Work out the finished part from the listing and answer in its coordinate system (mm). A direction names the side the tool comes from. Give positions to 0.01 mm unless a question says otherwise; leave off trailing zeros. Write each loop counter-clockwise with the first axis right and the second up, starting at its lowest first coordinate (ties: lowest second). Pieces come first, ordered by that corner, then holes.
1) Find section B-B (z = 3.75). Determine the outline of the cut face in (x, y), plus the area to 3 significant figures.
2) A tool of negligible diameter and unlimited length cuts with its end or side. For faces 1 (the face through (10, 19, 0)), 2 (the face through (-1, 31, 2)), 3 (the face through (-5, 34.5, 0)), 4 (the face through (-13, 3, 2)), from which of +Z, -Z, +X, -X, +Y, -Y can it reach the whole face along a straight path? Write none if from no direction.
3) Straight lines are drawn through the part: probe 1 along X at (y, z) = (28.5, 5.5); probe 2 along Y at (x, z) = (1.5, 0.5); probe 3 along Y at (x, z) = (3.5, 0.5). For each, find the intervals that lie inside material, in ascending order.
4) Determine the mould class of faces 5 (the face through (-18.719, -0.212, 0.826)), 6 (the face through (0, 12, 7)), 7 (the face through (-21, 0, 0)) for opening direction Z: pulls with the +Z half, pulls with the -Z half, needs draft (parallel to the pull), parting line crosses it, or undercut.
5) Given pin 1 Ø4 at (y, z) = (23.5, -0.5) entering from -X; pin 2 Ø4 at (x, z) = (15, -2) entering from +Y; pin 3 Ø5 at (y, z) = (15, -3.5) entering from +X, each flat-ended and moving along its own axis, determine where each tip first touches the part or whether it passes through.
6) Find section C-C (x = -1.5). Count the separate pieces of the cut face and the enclosed holes in it, plus the area to 3 significant figures.
7) Find section A-A (y = 20). Determine the outline of the cut face in (x, z).
8) Find section D-D (x = -12). Determine the outline of the cut face in (y, z).
```python
from build123d import *

# Parameters (mm, degrees)
BOSS_EXTRUDE1_DEPTH     = 7
SKETCH2_R               = 2.75
CUT_EXTRUDE1_DEPTH      = 39.5
CUT_EXTRUDE2_DEPTH      = 42.512046444
CUT_EXTRUDE2_DEPTH_BACK = 42.512046444
SKETCH5_R               = 2
CHAMFER2_SIZE           = 0.5
FILLET2_R               = 0.5


with BuildPart() as part:
    # Sketch1 → Boss-Extrude1 (new, symmetric)
    with BuildSketch(Plane.XY):
        with BuildLine():
            Line((-21, -3), (-21, 3))
            Line((-21, 3), (-10, 3))
            Line((-10, 3), (-10, 34.5))
            Line((-10, 34.5), (-1, 34.5))
            Line((-1, 34.5), (-1, 25.916079783))
            ThreePointArc((-1, 25.916079783), (0, 14), (1, 25.916079783))
            Line((1, 25.916079783), (1, 34.5))
            Line((1, 34.5), (10, 34.5))
            Line((10, 34.5), (10, 3))
            Line((10, 3), (21, 3))
            Line((21, 3), (21, -3))
            Line((21, -3), (-21, -3))
        make_face()
    extrude(amount=BOSS_EXTRUDE1_DEPTH, both=True)

    # Sketch2 → Cut-Extrude1 (cut, through all)
    with BuildSketch(Plane(origin=(0, 3, 0), x_dir=(1, 0, 0), z_dir=(0, 1, 0))):
        with Locations(Location((15.904501915, 0, 0), (0, 0, 180))):
            Circle(SKETCH2_R)
        with Locations(Location((-16.095498085, 0, 0), (0, 0, 180))):
            Circle(SKETCH2_R)
    extrude(amount=-CUT_EXTRUDE1_DEPTH, mode=Mode.SUBTRACT)

    # Sketch5 → Cut-Extrude2 (cut, two sides: drawn at the far end of the back side and taken through both)
    with BuildSketch(Plane(origin=(-1, 0, 0), x_dir=(0, 0, -1), z_dir=(1, 0, 0)).offset(-CUT_EXTRUDE2_DEPTH_BACK)):
        with Locations((0.330734984, 30.208039892)):
            Circle(SKETCH5_R)
    extrude(amount=CUT_EXTRUDE2_DEPTH + CUT_EXTRUDE2_DEPTH_BACK, mode=Mode.SUBTRACT)

    # Chamfer2
    chamfer2_edges = [part.edges().sort_by_distance(p)[0] for p in [
        (0, 14, -7),
        (0, 14, 7),
        (18.654501915, 3, 0),
        (-13.345498085, 3, 0),
        (-10, 30.208039892, 1.669265016),
        (10, 30.208039892, 1.669265016),
    ]]
    chamfer(chamfer2_edges, length=CHAMFER2_SIZE)

    # Fillet2
    fillet2_edges = [part.edges().sort_by_distance(p)[0] for p in [
        (-15.5, 3, 7),
        (10, 18.75, -7),
        (15.5, 3, -7),
        (-21, 0, 7),
        (21, 0, -7),
        (-21, 0, -7),
        (-15.5, 3, -7),
        (-10, 18.75, -7),
        (21, 0, 7),
        (10, 34.5, 0),
        (21, 3, 0),
        (21, -3, 0),
        (-21, -3, 0),
        (-21, 3, 0),
        (-10, 34.5, 0),
        (15.5, 3, 7),
        (10, 18.75, 7),
        (-10, 18.75, 7),
    ]]
    fillet(fillet2_edges, radius=FILLET2_R)


solid = part.part
```
Results:
1. outline: (-21, -2.5) arc R0.5 ccw to (-20.5, -3) - (20.5, -3) arc R0.5 ccw to (21, -2.5) - (21, 2.5) arc R0.5 ccw to (20.5, 3) - (10, 3) - (10, 34) arc R0.5 ccw to (9.5, 34.5) - (1, 34.5) - (1, 25.92) arc R6 cw (long way) to (-1, 25.92) - (-1, 34.5) - (-9.5, 34.5) arc R0.5 ccw to (-10, 34) - (-10, 3) - (-20.5, 3) arc R0.5 ccw to (-21, 2.5) - close
1. area: 752 mm2
2. face 1: +Z, -Z, +X, +Y
2. face 2: +Z, -Z, +Y
2. face 3: +Z, -Z, +X, -X, +Y
2. face 4: +Z, -Z, -X, +Y
3. probe 1: x = -10 to -1, 1 to 10
3. probe 2: y = -3 to 14.19, 25.81 to 28.39, 32.03 to 34.5
3. probe 3: y = -3 to 15.13, 24.87 to 28.39, 32.03 to 34.5
4. face 5: undercut
4. face 6: pulls with the +Z half
4. face 7: needs draft
5. pin 1: stops at x = -10
5. pin 2: stops at y = 3
5. pin 3: stops at x = 10
6. separate pieces: 2
6. enclosed holes: 1
6. area: 349 mm2
7. outline: (-10, -6.5) arc R0.5 ccw to (-9.5, -7) - (-6.5, -7) - (-6, -6.5) - (-6, 6.5) - (-6.5, 7) - (-9.5, 7) arc R0.5 ccw to (-10, 6.5) - close; (6, -6.5) - (6.5, -7) - (9.5, -7) arc R0.5 ccw to (10, -6.5) - (10, 6.5) arc R0.5 ccw to (9.5, 7) - (6.5, 7) - (6, 6.5) - close
8. outline: (-3, -7) - (2.5, -7) arc R0.5 ccw to (3, -6.5) - (3, 6.5) arc R0.5 ccw to (2.5, 7) - (-3, 7) - close
